Autodesk Inventor part; units mm, degrees
ref_plane "YZ Plane" through (0, 0, 0) normal (1, 0, 0) x (0, 1, 0)
ref_plane "XZ Plane" through (0, 0, 0) normal (0, 1, 0) x (-1, 0, 0)
ref_plane "XY Plane" through (0, 0, 0) normal (0, 0, 1) x (1, 0, 0)
sketch "Sketch1" plane through (0, 0, 0) normal (0, 1, 0) x (-1, 0, 0)
  circle A0 centre (0, 0) radius 1.5
  line L0 (0, 0) -> (0, -35) construction
  circle A1 centre (0, -35) radius 1.5
  circle A2 centre (0, 0) radius 4.5
  circle A3 centre (0, -35) radius 4.5
  line L1 (4.5, 0) -> (4.5, -35)
  line L2 (-4.5, -35) -> (-4.5, 0)
  dimension "d0" = 3
  dimension "d1" = 3
  dimension "d2" = 3
  dimension "d3" = 3
  dimension "d4" = 35
extrude "Extrusion1" add sketch "Sketch1" along normal mid plane 3
properties part number "barras_micro"
Part model, mm, in its own coordinate system. Coordinates: 2 decimals unless noted, no trailing zeros. Order: outer loops, then holes, each group sorted by start corner. A loop starts at its lowest first (then second) coordinate and runs counter-clockwise, first axis right, second up. Notation, with made-up numbers: M 62.25,32.5 L 85.25,32.5 A17 cw 85.25,61.5 Z; hole C 84.25,-14.75 d2. An arc over 180 degrees is marked long. Use a Markdown table: item, result.
(1) Cut at A-A on x = 0. Write the cut outline in (y, z).
A:
| item | result |
|---|---|
| outline | M -1.5,-39.5 L 1.5,-39.5 L 1.5,-36.5 L -1.5,-36.5 Z; M -1.5,-33.5 L 1.5,-33.5 L 1.5,-1.5 L -1.5,-1.5 Z; M -1.5,1.5 L 1.5,1.5 L 1.5,4.5 L -1.5,4.5 Z |
(2) Probe L1, parallel to Z at x = 0, y = -0.95; L2, parallel to Z at x = -2.25, y = -1.15; L3, parallel to Z at x = 2.5, y = -0.3. List the from-to ranges inside material, lowest first.
A:
| item | result |
|---|---|
| L1 | z = -39.5 to -36.5, -33.5 to -1.5, 1.5 to 4.5 |
| L2 | z = -38.9 to 3.9 |
| L3 | z = -38.74 to 3.74 |
(3) Cut at C-C on z = -35.5. Write the cut outline in (x, y).
A:
| item | result |
|---|---|
| outline | M -4.47,-1.5 L -1.41,-1.5 L -1.41,1.5 L -4.47,1.5 Z; M 1.41,-1.5 L 4.47,-1.5 L 4.47,1.5 L 1.41,1.5 Z |
(4) Flat gauge pin, fed straight in: pin 1 (1.5 mm diameter, centred on x = 1, y = 1, fed in from +Z). Where does the tip first touch, or does it go through?
A:
| item | result |
|---|---|
| pin 1 | stops at z = 4.49 |
(5) Pull direction Z, two halves, no side cores. Call faces 1 (the cylindrical face through (-0.1, 0, -39.5)), 2 (the cylindrical face through (0.1, 0, 4.5)), 3 (the flat face through (0, 1.5, -17)), 4 (the cylindrical face through (1.5, -0.02, -0.07)): released by +Z, released by -Z, zero draft, split by the parting line, or undercut.
A:
| item | result |
|---|---|
| face 1 | released by -Z |
| face 2 | released by +Z |
| face 3 | zero draft |
| face 4 | undercut |
(6) Cut at B-B on y = 0.2. Write the cut outline in (x, z).
A:
| item | result |
|---|---|
| outline | M -4.5,-35 A4.5 ccw 4.5,-35 L 4.5,0 A4.5 ccw -4.5,0 Z; hole C 0,-35 d3; hole C 0,0 d3 |
(7) Cut at D-D on x = 2.5. Write the cut outline in (y, z).
A:
| item | result |
|---|---|
| outline | M -1.5,-38.74 L 1.5,-38.74 L 1.5,3.74 L -1.5,3.74 Z |
